Geometry: see drawing. Coordinates: mm, zero at the bounding-box minimum. A direction names the side the tool comes from. Coordinates: 2 decimals unless noted, no trailing zeros. Order: outer loops, then holes, each group sorted by start corner. A loop starts at its lowest first (then second) coordinate and runs counter-clockwise, first axis right, second up.
Item 1: Ray query, line 1 (X direction, y = 7.5, z = 27); line 2 (Y direction, x = 119.5, z = 53.5); line 3 (X direction, y = 23.5, z = 20.5). Return the intervals inside material, ascending.
Item 2: Reachability of the marked faces 1, 2 and 3 from +Z, -Z, +X, -X, +Y, -Y: full face, straight path, thin tool, end or side. Return the list, or none.
Item 3: Contact query for flat-ended pins moving along their axis: P1, Ø3, axis at x = 80.5, y = 7, coming from the +Z side; P2, Ø4, axis at y = 95, z = 21.5, coming from the +X side; P3, Ø3, axis at x = 52, z = 13.5, coming from the -Y side. Output: stop coordinate, or through.
Item 4: Section C-C on x = 59.5. Return the cut outline in (y, z) (3 decimals).
Item 5: Section B-B on y = 80. Return the cut outline in (x, z), then the cut area to 3 significant figures.
Item 6: Section A-A on z = 13.5. Return the cut outline in (x, y), then the cut area to 3 significant figures.
Item 7: Section D-D on x = 11.5. Return the cut outline in (y, z) (3 decimals), then the cut area to 3 significant figures.
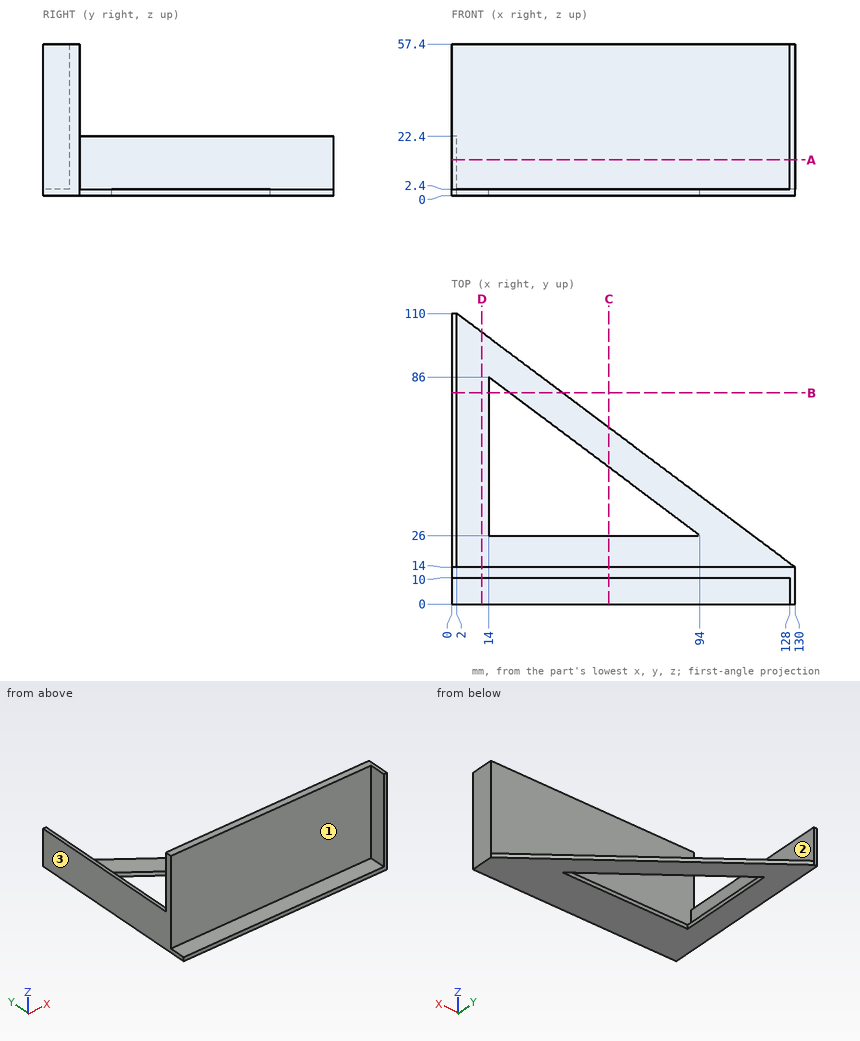
Answer list:
1. line 1: x = 128 to 130
1. line 2: y = 10 to 14
1. line 3: x = 0 to 2
2. face 1: +Z, -X, -Y
2. face 2: +Z, +X, +Y
2. face 3: +Z, -Z, -X, +Y, -Y
3. P1: stops at z = 2.4
3. P2: stops at x = 2
3. P3: stops at y = 10
4. outline: (0, 0) - (26, 0) - (26, 2.4) - (14, 2.4) - (14, 57.4) - (10, 57.4) - (10, 2.4) - (0, 2.4) - close; (51.875, 0) - (66.875, 0) - (66.875, 2.4) - (51.875, 2.4) - close
5. outline: (0, 0) - (14, 0) - (14, 2.4) - (2, 2.4) - (2, 22.4) - (0, 22.4) - close; (22, 0) - (42, 0) - (42, 2.4) - (22, 2.4) - close
5. area: 122 mm2
6. outline: (0, 10) - (128, 10) - (128, 0) - (130, 0) - (130, 14) - (2, 14) - (2, 110) - (0, 110) - close
6. area: 732 mm2
7. outline: (0, 0) - (102.875, 0) - (102.875, 2.4) - (14, 2.4) - (14, 57.4) - (10, 57.4) - (10, 2.4) - (0, 2.4) - close
7. area: 467 mm2
